Input: part model. Units: mm. Frame: model coordinates. A direction names the side the tool comes from. Give positions to 0.01 mm unless a question says otherwise; leave off trailing zeros. Loops run counter-clockwise (first coordinate to the right, second up) from the corner with the lowest first, then second, coordinate; pieces in that order, holes last. Notation, with made-up numbers: M 80,63.5 L 88,63.5 A18 ccw 88,74.5 Z; hole C 34.5,33.5 d4. An arc over 180 degrees is marked long. Answer as a JSON object with one key per item and string values. Group by question number.
1) First-contact query: P1, Ø1.6, axis at y = -1, z = 51.5, coming from the +X side; P2, Ø5, axis at x = 25.4, z = -38.1, coming from the -Y side (3 decimals); P3, Ø3.5, axis at x = -12.7, z = -50.8, coming from the +Y side. Flat tips, straight axial feed; report the tip coordinate or a pass-through.
2) Access query for faces 1 (the flat face through (-25.4, -2, 53)), 2 (the cylindrical face through (14.396, -1.61, -22.341)), 3 (the flat face through (63.5, -2, -45)). Directions: +Z, -Z, +X, -X, +Y, -Y. A direction counts if a zero-diameter tool reaches every point of the face in a straight line with its end or side. Return the directions, or none.
3) Section query C-C on x = 50.5. Return loops of the section in (y, z) (3 decimals), plus the area to 4 significant figures.
4) Section query A-A on z = 50.8. Return loops of the section in (x, y) (3 decimals).
5) Draft query along Z for faces 4 (the flat face through (-63.5, -2, 1)), 5 (the cylindrical face through (-49.02, -1.57, -14.07)), 6 (the flat face through (-25.4, -2, -6)). Return one class per face: +Z half, -Z half, draft (parallel to the pull), parting line (faces both ways), or undercut.
6) Section query D-D on y = -1.5. Count the separate pieces of the cut face and the enclosed holes in it, plus the area to 3 significant figures.
7) Ray query, L1, parallel to Z at x = 50.8, y = -2.5 (3 decimals); L2, parallel to X at y = -0.8, z = -11.5; L3, parallel to X at y = -1, z = -37. Return the intervals inside material, ascending.
8) Section query B-B on x = 25.4. Return loops of the section in (y, z) (3 decimals).
from build123d import *

# Parameters (mm, degrees)
F1_DEPTH = 3.175
F2_R     = 3.175
F3_R     = 5.08
F5_D     = 6.35
F6_D     = 4.4958


with BuildPart() as f1:
    # F0 (on Front) → F1 (new body)
    with BuildSketch(Plane.XZ):
        Polygon((-25.4, 63.5), (-63.5, 63.5), (-63.5, -63.5), (63.5, -63.5), (63.5, -25.4), (44.45, -25.4), (-25.4, 44.45), align=None)
        Polygon((-25.4, -25.4), (-25.4, 21.99936), (21.99936, -25.4), align=None, mode=Mode.SUBTRACT)
    extrude(amount=F1_DEPTH)

    # F2
    f2_edges = [f1.edges().sort_by_distance(p)[0] for p in [
        (-25.4, -1.5875, 63.5),
        (-25.4, -1.5875, 44.45),
        (44.45, -1.5875, -25.4),
        (63.5, -1.5875, -25.4),
        (63.5, -1.5875, -63.5),
        (-63.5, -1.5875, -63.5),
        (-63.5, -1.5875, 63.5),
    ]]
    fillet(f2_edges, radius=F2_R)

    # F3
    f3_edges = [f1.edges().sort_by_distance(p)[0] for p in [
        (21.99936, -1.5875, -25.4),
        (-25.4, -1.5875, -25.4),
        (-25.4, -1.5875, 21.99936),
    ]]
    fillet(f3_edges, radius=F3_R)

    # F5 (through all)
    with Locations(Plane.XZ.offset(3.175)):
        with Locations((-50.8, 50.8), (-50.8, -25.4), (50.8, -50.8), (-25.4, -50.8)):
            Hole(F5_D / 2)

    # F6 (through all)
    with Locations(Plane.XZ.offset(3.175)):
        with Locations((-50.8, 38.1), (-38.1, 50.8), (-38.1, 25.4), (-50.8, 12.7), (-38.1, 0), (-50.8, -12.7), (-38.1, -38.1), (-50.8, -38.1), (-50.8, -50.8), (-38.1, -50.8), (-12.7, -50.8), (0, -38.1), (12.7, -50.8), (25.4, -38.1), (38.1, -50.8), (50.8, -38.1)):
            Hole(F6_D / 2)


solid = f1.part
Output:
{
 "1": {"P1": "stops at x = -25.4", "P2": "stops at y = -3.175", "P3": "passes through"},
 "2": {"face 1": "+Z, +X, +Y, -Y", "face 2": "+Y, -Y", "face 3": "+Z, -Z, +X, +Y, -Y"},
 "3": {"outline": "M -3.175,-63.5 L 0,-63.5 L 0,-53.961 L -3.175,-53.961 Z; M -3.175,-47.639 L 0,-47.639 L 0,-40.328 L -3.175,-40.328 Z; M -3.175,-35.872 L 0,-35.872 L 0,-25.4 L -3.175,-25.4 Z", "area": "86.75 mm^2"},
 "4": {"outline": "M -63.5,-3.175 L -53.975,-3.175 L -53.975,0 L -63.5,0 Z; M -47.625,-3.175 L -40.348,-3.175 L -40.348,0 L -47.625,0 Z; M -35.852,-3.175 L -25.4,-3.175 L -25.4,0 L -35.852,0 Z"},
 "5": {"face 4": "draft", "face 5": "undercut", "face 6": "undercut"},
 "6": {"separate pieces": "1", "enclosed holes": "21", "area": "9,220 mm^2"},
 "7": {"L1": "z = -63.5 to -53.975, -47.625 to -40.348, -35.852 to -25.4", "L2": "x = -63.5 to -52.7, -48.9 to -25.4, 8.1 to 30.55", "L3": "x = -63.5 to -52.76, -48.84 to -40.06, -36.14 to -1.96, 1.96 to 23.44, 27.36 to 48.84, 52.76 to 63.5"},
 "8": {"outline": "M -3.175,-63.5 L 0,-63.5 L 0,-40.348 L -3.175,-40.348 Z; M -3.175,-35.852 L 0,-35.852 L 0,-6.35 L -3.175,-6.35 Z"}
}
